Source: CAD feature listing. Evaluate the final solid. Frame: model axes, mm. A direction names the side the tool comes from. Coordinates: 2 decimals unless noted, no trailing zeros. Loops run counter-clockwise (first coordinate to the right, second up) from the corner with the lowest first, then second, coordinate; pieces in that order, holes last. Notation, with made-up numbers: M 27.5,-10 L 33.5,-10 A12 ccw 33.5,4 Z; hole C 14.5,3.5 d1. An arc over 180 degrees is marked long. One line per question, with ' | ' between items. Start each with the question number.
1. Section query A-A, the plane z = 30.5. Output: boundary loops of the cut face in (x, y), and give its area (3 significant figures).
2. Section query D-D, the plane y = 0. Output: boundary loops of the cut face in (x, z).
3. Access query for faces 1 (the flat face through (4, -4, 3)), 2 (the flat face through (2.2, -0.1, 36)). Directions: +Z, -Z, +X, -X, +Y, -Y. A direction counts if a zero-diameter tool reaches every point of the face in a straight line with its end or side. Return the directions, or none.
4. Mould query, pull axis Y, two halves, no side actions, for faces 3 (the cylindrical face through (4.88, -1.08, 20.79)), 4 (the flat face through (0, 5, 4)), 5 (the flat face through (-1.85, 0, 32)). Classes: pulls with the +Y half, pulls with the -Y half, needs draft (parallel to the pull), parting line crosses it, or undercut.
5. Ray query, probe 1 along Y at (x, z) = (0, 1.3) (3 decimals); probe 2 along Z at (x, y) = (-2.5, 5); probe 3 along Z at (x, y) = (-1.75, 4.75). Return the intervals inside material, ascending.
6. Pin query (flat end, axial travel): P1, Ø1, axis at x = 4, z = 11.5, coming from the -Y side; P2, Ø2, axis at y = 5.5, z = 29, coming from the +X side; P3, Ø5, axis at y = 1.5, z = 20, coming from the -X side. Return the tip coordinate at first contact, or that it passes through.
7. Section query C-C, the plane y = 6.5. Output: boundary loops of the cut face in (x, z), and give its area (3 significant figures).
8. Section query B-B, the plane x = 1.25. Output: boundary loops of the cut face in (y, z), and give its area (3 significant figures).
```python
from build123d import *

# Parameters (mm, degrees)
SKETCH1_R           = 10
SKETCH1_R_2         = 1.625
BOSS_EXTRUDE1_DEPTH = 3
BOSS_EXTRUDE2_DEPTH = 3
SKETCH3_R           = 5
BOSS_EXTRUDE3_DEPTH = 30
CUT_EXTRUDE1_DEPTH  = 8


with BuildPart() as part:
    # Sketch1 → Boss-Extrude1 (new body)
    with BuildSketch(Plane.XY):
        Circle(SKETCH1_R)
        with Locations((0, 7)):
            Circle(SKETCH1_R_2, mode=Mode.SUBTRACT)
    extrude(amount=BOSS_EXTRUDE1_DEPTH)

    # Sketch2 → Boss-Extrude2 (add)
    with BuildSketch(Plane.XY.offset(3)):
        with BuildLine():
            Line((-2.291287847, 5), (2.291287847, 5))
            ThreePointArc((2.291287847, 5), (0, -5.5), (-2.291287847, 5))
        make_face()
    extrude(amount=BOSS_EXTRUDE2_DEPTH)

    # Sketch3 → Boss-Extrude3 (add)
    with BuildSketch(Plane.XY.offset(6)):
        with Locations(Location((0, 0, 0), (0, 0, 90))):
            Circle(SKETCH3_R)
    extrude(amount=BOSS_EXTRUDE3_DEPTH)

    # Sketch4 → Cut-Extrude1 (cut)
    with BuildSketch(Plane.XY.offset(36)):
        with BuildLine():
            Line((1.85, -1.966596044), (1.85, 1.966596044))
            ThreePointArc((1.85, 1.966596044), (0, 2.7), (-1.85, 1.966596044))
            Line((-1.85, 1.966596044), (-1.85, -1.966596044))
            ThreePointArc((-1.85, -1.966596044), (0, -2.7), (1.85, -1.966596044))
        make_face()
    extrude(amount=-CUT_EXTRUDE1_DEPTH, mode=Mode.SUBTRACT)


solid = part.part
```
Taken from the geometry:
1) outline: C 0,0 d10; hole M -1.85,-1.97 A2.7 ccw 1.85,-1.97 L 1.85,1.97 A2.7 ccw -1.85,1.97 Z | area: 60.3 mm^2
2) outline: M -10,0 L 10,0 L 10,3 L 5.5,3 L 5.5,6 L 5,6 L 5,36 L 1.85,36 L 1.85,28 L -1.85,28 L -1.85,36 L -5,36 L -5,6 L -5.5,6 L -5.5,3 L -10,3 Z
3) face 1: +Z | face 2: +Z, +X, -X, +Y, -Y
4) face 3: parting line crosses it | face 4: pulls with the +Y half | face 5: undercut
5) probe 1: -10 to 5.375, 8.625 to 10 | probe 2: 0 to 3 | probe 3: 0 to 6
6) P1: y = -3.57 | P2: x = 2.18 | P3: x = -5
7) outline: M -7.6,0 L -1.55,0 L -1.55,3 L -7.6,3 Z; M 1.55,0 L 7.6,0 L 7.6,3 L 1.55,3 Z | area: 36.3 mm^2
8) outline: M -9.92,0 L 5.96,0 L 5.96,3 L 5,3 L 5,6 L 4.84,6 L 4.84,36 L 2.39,36 L 2.39,28 L -2.39,28 L -2.39,36 L -4.84,36 L -4.84,6 L -5.36,6 L -5.36,3 L -9.92,3 Z; M 8.04,0 L 9.92,0 L 9.92,3 L 8.04,3 Z | area: 337 mm^2
